Can you work these out from the drawing? Everything is in mm from the part's minimum corner. Round coordinates to 2 decimals unless told otherwise and drop trailing zeros. Write each loop counter-clockwise with the first axis right and the second up, starting at its lowest first coordinate (ties: lowest second). Pieces come first, ordered by that corner, then holes. Notation, with made-up numbers: M -33.5,-33 L 18.5,-33 A18 ccw 18.5,-9 Z; hole C 24,77 d7. An arc over 180 degrees is marked long. Answer in a Markdown table with one row per item. Add a question column.
(1) If I drill on probe 1 along Z at (x, y) = (29, 101) (1 decimal); probe 2 along Z at (x, y) = (14, 151.5) (1 decimal); probe 3 along Z at (x, y) = (18, 12.5) (1 decimal), over which ranges is the centre line in solid material (lowest first)?
(2) Suppose I cut it at B-B, the plane x = 12.5. Write out the boundary of the cut face in (y, z) (1 decimal).
(3) Suppose I cut it at A-A, the plane y = 180. Count the separate pieces of the cut face and the enclosed holes in it, then the cut area to 3 significant figures.
(4) Suppose I cut it at D-D, the plane z = 380.5. Write out the boundary of the cut face in (x, y), then the cut area to 3 significant figures.
(5) Suppose I cut it at C-C, the plane y = 142. Write out the boundary of the cut face in (x, z) (1 decimal), then the cut area to 3 significant figures.
(6) I'm going to push flat-ended pins straight in: pin 1 (8 mm diameter, centred on x = 29.5, y = 126.5, fed in from +Z); pin 2 (12 mm diameter, centred on x = 7.5, z = 114, fed in from -Y); pin 3 (6 mm diameter, centred on x = 22.5, y = 172.5, fed in from -Z). Where does each tip first touch, or does it pass through?
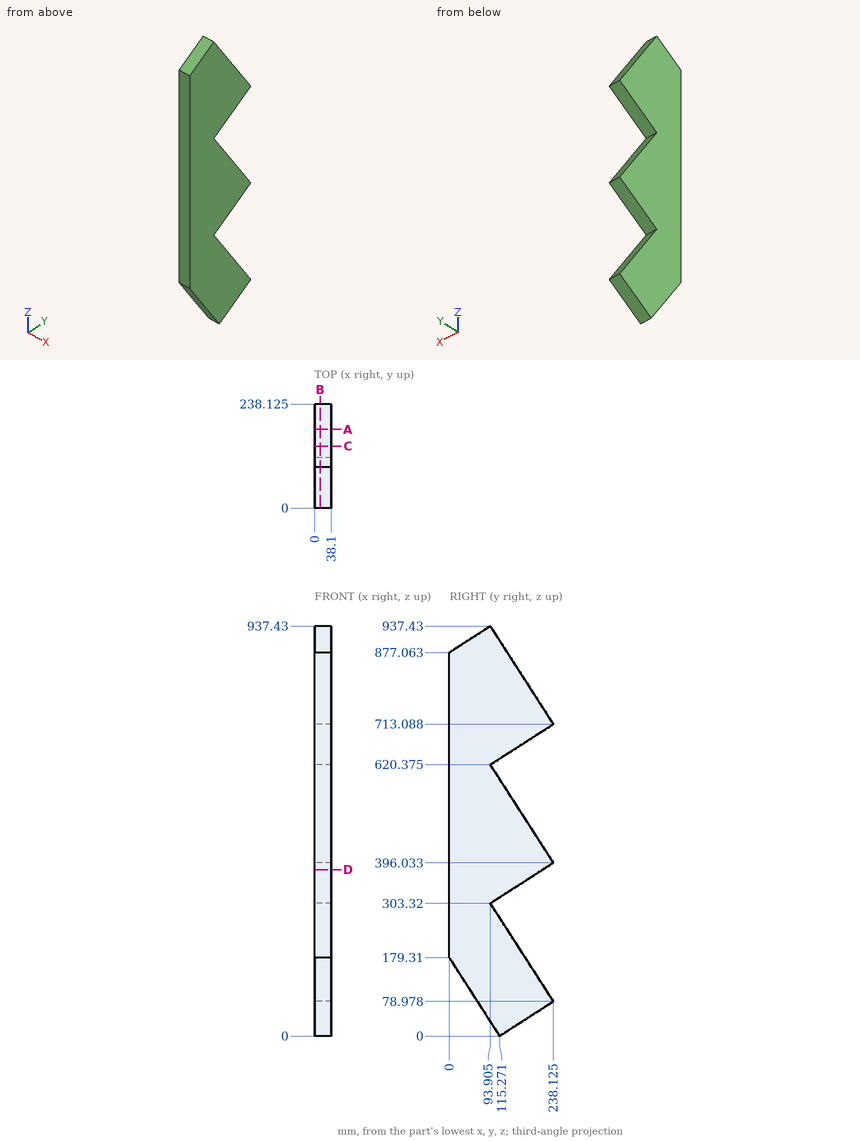
Calculated:
| question | item | result |
|---|---|---|
| 1 | probe 1 | 22.2 to 292.3, 307.9 to 609.3, 624.9 to 926.4 |
| 1 | probe 2 | 23.3 to 213.7, 340.3 to 530.8, 657.4 to 847.8 |
| 1 | probe 3 | 159.9 to 885.1 |
| 2 | outline | M 0,179.3 L 115.3,0 L 238.1,79 L 93.9,303.3 L 238.1,396 L 93.9,620.4 L 238.1,713.1 L 93.9,937.4 L 0,877.1 Z |
| 3 | separate pieces | 3 |
| 3 | enclosed holes | 0 |
| 3 | area | 14,600 mm² |
| 4 | outline | M 0,0 L 38.1,0 L 38.1,213.96 L 0,213.96 Z |
| 4 | area | 8,150 mm² |
| 5 | outline | M 0,17.2 L 38.1,17.2 L 38.1,228.5 L 0,228.5 Z; M 0,334.2 L 38.1,334.2 L 38.1,545.6 L 0,545.6 Z; M 0,651.3 L 38.1,651.3 L 38.1,862.6 L 0,862.6 Z |
| 5 | area | 24,200 mm² |
| 6 | pin 1 | z = 892.95 |
| 6 | pin 2 | y = 38.13 |
| 6 | pin 3 | z = 34.86 |
